Design review of the part built by this model. Coordinates are the model's own, in mm. A direction names the side the tool comes from. Round coordinates to 2 decimals unless told otherwise and drop trailing zeros. Write each loop counter-clockwise with the first axis right and the second up, starting at its lowest first coordinate (ties: lowest second). Pieces come first, ordered by that corner, then holes. Notation, with made-up numbers: M 31,16 L 63,16 A18 cw 63,50 Z; hole C 70.5,32.25 d5. An arc over 180 degrees is marked long. Use CSV: the item, a comma, the result in double quotes.
from build123d import *

# Parameters (mm, degrees)
SKETCH1_W           = 16.6
SKETCH1_H           = 24
BOSS_EXTRUDE1_DEPTH = 10


with BuildPart() as part:
    # Sketch1 → Boss-Extrude1 (new body)
    with BuildSketch(Plane.XY):
        Rectangle(SKETCH1_W, SKETCH1_H)
        Polygon((-4.9, 10), (-4.9, 0.65), (4.9, 0.65), (4.9, 10), (6.3, 10), (6.3, -10), (4.9, -10), (4.9, -0.65), (-4.9, -0.65), (-4.9, -10), (-6.3, -10), (-6.3, 10), align=None, mode=Mode.SUBTRACT)
    extrude(amount=BOSS_EXTRUDE1_DEPTH)


solid = part.part
1) The part is to be moulded in two halves that separate along X. For faces 1 (the face through (-8.3, 0, 5)), 2 (the face through (8.3, 0, 5)), 3 (the face through (-6, -10, 5)), say which applies: released by +X, released by -X, zero draft, split by the parting line, or undercut.
Answers:
face 1,"released by -X"
face 2,"released by +X"
face 3,"undercut"
2) For pin 1 Ø3 at (x, y) = (6, 2.5) entering from +Z, flat-tipped, find the tip position at first contact; note if it passes through.
Answers:
pin 1,"z = 10"
3) Wall thickness on line 1 along X through (y, z) = (-4.75, 0.5); line 2 along Y through (x, z) = (4, 9.25); line 3 along Y through (x, z) = (-5, 1): over which ranges is each line inside the solid? List them lowest first. Write a range as [from, to].
Answers:
line 1,"[-8.3, -6.3], [-4.9, 4.9], [6.3, 8.3]"
line 2,"[-12, -0.65], [0.65, 12]"
line 3,"[-12, -10], [10, 12]"
4) Add section C-C on x = -4. Write out the cut boundary in (y, z).
Answers:
outline,"M -12,0 L -0.65,0 L -0.65,10 L -12,10 Z; M 0.65,0 L 12,0 L 12,10 L 0.65,10 Z"
5) Machinability: for faces 4 (the face through (0, 3, 10)), 5 (the face through (6, -10, 5)), which of the approach directions +Z, -Z, +X, -X, +Y, -Y give a long, thin tool a straight path to every point of the face, cutting with its end or side? Answer none if there is none.
Answers:
face 4,"+Z, +X, -X, +Y, -Y"
face 5,"+Z, -Z"
6) Add section A-A on y = -2. Write out the cut boundary in (x, z), then the cut area to 3 significant figures.
Answers:
outline,"M -8.3,0 L -6.3,0 L -6.3,10 L -8.3,10 Z; M -4.9,0 L 4.9,0 L 4.9,10 L -4.9,10 Z; M 6.3,0 L 8.3,0 L 8.3,10 L 6.3,10 Z"
area,"138 mm²"
7) Add section B-B on z = 9.75. Write out the cut boundary in (x, y).
Answers:
outline,"M -8.3,-12 L 8.3,-12 L 8.3,12 L -8.3,12 Z; hole M -6.3,-10 L -4.9,-10 L -4.9,-0.65 L 4.9,-0.65 L 4.9,-10 L 6.3,-10 L 6.3,10 L 4.9,10 L 4.9,0.65 L -4.9,0.65 L -4.9,10 L -6.3,10 Z"
